Autodesk Inventor part; units mm, degrees
ref_plane "YZ Plane" through (0, 0, 0) normal (1, 0, 0) x (0, 1, 0)
ref_plane "XZ Plane" through (0, 0, 0) normal (0, 1, 0) x (-1, 0, 0)
ref_plane "XY Plane" through (0, 0, 0) normal (0, 0, 1) x (1, 0, 0)
sketch "草圖1" plane through (0, 0, 0) normal (0, 1, 0) x (-1, 0, 0)
  circle A0 centre (0, 0) radius 25
  line L0 (25, 0) -> (-25, 0)
  line L1 (-25, 0) -> (-25, -25)
  line L2 (-25, -25) -> (25, -25)
  line L3 (25, -25) -> (25, 0)
  dimension "d0" = 50
extrude "擠出1" add sketch "草圖1" along normal mid plane 3
sketch "草圖2" plane through (0, 1.5, 0) normal (0, 1, 0) x (1, 0, 0)
  line L0 (-25, 25) -> (-25, 0)
  line L1 (25, 0) -> (25, 25)
  line L2 (-25, 25) -> (25, 25)
  line L3 (25, 25) -> (25, 22)
  line L4 (25, 22) -> (-25, 22)
  line L5 (-25, 22) -> (-25, 25)
  point P0 (0, 0)
  dimension "d3" = 3
extrude "擠出2" add sketch "草圖2" along normal blind 50
sketch "草圖3" plane through (-25, 1.5, -22) normal (0, 0, 1) x (1, 0, 0)
  circle A0 centre (25, 25) radius 25
  line L0 (0, 50) -> (50, 50)
  line L1 (50, 0) -> (50, 50)
  line L2 (50, 0) -> (0, 0)
  line L3 (50, 0) -> (50, 50)
  line L4 (0, 50) -> (50, 50)
  line L5 (0, 0) -> (0, 50)
  point P0 (25, -1.5)
  point P1 (25, 50)
  point P2 (0, 25)
  point P3 (50, 25)
extrude "擠出3" cut sketch "草圖3" against normal up to surface (3 mm away) contours A0 L0 L1 | A0 L5 L0
properties part number "Base_1"
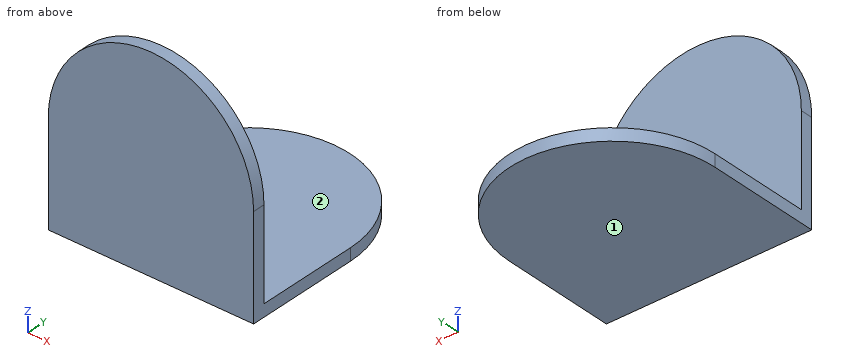
Work out the finished part from the listing and answer in its coordinate system (mm). Face numbers are marked on the shaded views. A direction names the side the tool comes from. Give positions to 0.01 mm unless a question says otherwise; leave off trailing zeros. Loops run counter-clockwise (first coordinate to the right, second up) from the corner with the lowest first, then second, coordinate; pieces in that order, holes last. Notation, with made-up numbers: (-6, 40) -> (6, 40) arc R29 cw to (6, 79) -> close; hole circle Ø6 at (-10, 27). An arc over 180 degrees is marked (long way). Use a Markdown table: item, result. Add a question column.
1. Section D-D on x = 21.5 is taken. Determine the outline of the cut face in (y, z).
2. A flat-ended cylindrical pin translates along its axis: pin 1 Ø1.5 at (x, z) = (5, 10.5) entering from +Y. Find the tip coordinate at first contact, or state that the pin passes through.
3. Section C-C on y = 41.5 is taken. Determine the outline of the cut face in (x, z), and give its area (3 significant figures).
4. Section B-B on z = -18 is taken. Determine the outline of the cut face in (x, y), and give its area (3 significant figures).
5. For the marked faces 1 and 2, determine the directions among +Z, -Z, +X, -X, +Y, -Y from which every point of the face is accessible in a straight line to the end or side of a thin tool.
6. Find the intervals of material crossed by probe 1 along Z at (x, y) = (-9.5, 42.5); probe 2 along Y at (x, z) = (-7.5, 3), in increasing order.
7. Section A-A on x = 0 is taken. Determine the outline of the cut face in (y, z), and give its area (3 significant figures).
Results below:
| question | item | result |
|---|---|---|
| 1 | outline | (-1.5, -25) -> (39.26, -25) -> (39.26, -22) -> (1.5, -22) -> (1.5, 12.76) -> (-1.5, 12.76) -> close |
| 2 | pin 1 | stops at y = 1.5 |
| 3 | outline | (-20, -25) -> (20, -25) -> (20, -22) -> (-20, -22) -> close |
| 3 | area | 120 mm^2 |
| 4 | outline | (-25, -1.5) -> (25, -1.5) -> (25, 1.5) -> (-25, 1.5) -> close |
| 4 | area | 150 mm^2 |
| 5 | face 1 | -Z, +X, -X, +Y, -Y |
| 5 | face 2 | +Z, +X, -X, +Y |
| 6 | probe 1 | z = -25 to -22 |
| 6 | probe 2 | y = -1.5 to 1.5 |
| 7 | outline | (-1.5, -25) -> (51.5, -25) -> (51.5, -22) -> (1.5, -22) -> (1.5, 25) -> (-1.5, 25) -> close |
| 7 | area | 300 mm^2 |
